```python
from build123d import *

# Parameters (mm, degrees)
SKETCH_1_R          = 2.025
SKETCH_1_R_2        = 13.1
SKETCH_1_R_3        = 3
EXTRUDE_1_DEPTH     = 5
SKETCH_3_R          = 24
CUT_EXTRUDE_2_DEPTH = 10
CUT_EXTRUDE_3_DEPTH = 10
FILLET_1_R          = 3
SKETCH_7_R          = 1.525
CUT_EXTRUDE_4_DEPTH = 10


with BuildPart() as part:
    # 草图1 → 凸台-拉伸1 (new body)
    with BuildSketch(Plane(origin=(0, 0, 0), x_dir=(1, 0, 0), z_dir=(0, 1, 0))):
        with BuildLine():
            Line((76.972140647, 43.13107423), (-4.193547259, 32.732463418))
            ThreePointArc((-4.193547259, 32.732463418), (-32.337515252, -6.579141836), (8.929411765, -31.768940894))
            Line((8.929411765, -31.768940894), (87.705882353, -9.626951786))
            ThreePointArc((87.705882353, -9.626951786), (94.014523475, -4.328783491), (94.205048973, 3.907310252))
            ThreePointArc((94.205048973, 3.907310252), (89.748559809, 18.25955029), (88.242912543, 33.212145922))
            ThreePointArc((88.242912543, 33.212145922), (84.849435117, 40.719066694), (76.972140647, 43.13107423))
        make_face()
        with Locations((0, 17.5)):
            Circle(SKETCH_1_R, mode=Mode.SUBTRACT)
        with Locations((8.75, 15.155444566)):
            Circle(SKETCH_1_R, mode=Mode.SUBTRACT)
        with Locations((-8.75, -15.155444566)):
            Circle(SKETCH_1_R, mode=Mode.SUBTRACT)
        with Locations((0, -17.5)):
            Circle(SKETCH_1_R, mode=Mode.SUBTRACT)
        with Locations((-15.155444566, -8.75)):
            Circle(SKETCH_1_R, mode=Mode.SUBTRACT)
        with Locations((8.75, -15.155444566)):
            Circle(SKETCH_1_R, mode=Mode.SUBTRACT)
        with Locations((15.155444566, -8.75)):
            Circle(SKETCH_1_R, mode=Mode.SUBTRACT)
        with Locations((-17.5, 0)):
            Circle(SKETCH_1_R, mode=Mode.SUBTRACT)
        Circle(SKETCH_1_R_2, mode=Mode.SUBTRACT)
        with Locations((-15.155444566, 8.75)):
            Circle(SKETCH_1_R, mode=Mode.SUBTRACT)
        with Locations((17.5, 0)):
            Circle(SKETCH_1_R, mode=Mode.SUBTRACT)
        with Locations((15.155444566, 8.75)):
            Circle(SKETCH_1_R, mode=Mode.SUBTRACT)
        with Locations((-8.75, 15.155444566)):
            Circle(SKETCH_1_R, mode=Mode.SUBTRACT)
        with Locations((85, 0)):
            Circle(SKETCH_1_R_3, mode=Mode.SUBTRACT)
        with Locations((78.242912543, 33.212145922)):
            Circle(SKETCH_1_R_3, mode=Mode.SUBTRACT)
    extrude(amount=EXTRUDE_1_DEPTH)

    # 草图3 → 切除-拉伸2 (cut)
    with BuildSketch(Plane(origin=(0, 5, 0), x_dir=(1, 0, 0), z_dir=(0, 1, 0))):
        Circle(SKETCH_3_R)
    extrude(amount=-CUT_EXTRUDE_2_DEPTH, mode=Mode.SUBTRACT)

    # 草图4 → 切除-拉伸3 (cut)
    with BuildSketch(Plane(origin=(0, 5, 0), x_dir=(1, 0, 0), z_dir=(0, 1, 0))):
        Polygon((69.770383541, 34.143027562), (75.881597407, 4.105451761), (16.636114037, 27.335685646), align=None)
        with BuildLine():
            ThreePointArc((32, 0), (30.461655113, -9.802426627), (25.994527014, -18.662383699))
            Line((25.994527014, -18.662383699), (76.108728609, -4.576602785))
            Line((76.108728609, -4.576602785), (28.785186198, 13.979021981))
            ThreePointArc((28.785186198, 13.979021981), (31.185942012, 7.171960739), (32, 0))
        make_face()
    extrude(amount=-CUT_EXTRUDE_3_DEPTH, mode=Mode.SUBTRACT)

    # 圆角1
    fillet_1_edges = [part.edges().sort_by_distance(p)[0] for p in [
        (25.994527014, 2.5, 18.662383699),
        (28.785186198, 2.5, -13.979021981),
        (76.108728609, 2.5, 4.576602785),
        (69.770383541, 2.5, -34.143027562),
        (75.881597407, 2.5, -4.105451761),
        (16.636114037, 2.5, -27.335685646),
    ]]
    fillet(fillet_1_edges, radius=FILLET_1_R)

    # 草图7 → 切除-拉伸4 (cut)
    with BuildSketch(Plane.XZ):
        with Locations((0, -27.522163408)):
            Circle(SKETCH_7_R)
        with Locations((33.321534862, -16.496811603)):
            Circle(SKETCH_7_R)
        with Locations((-27.522163408, 0)):
            Circle(SKETCH_7_R)
        with Locations((0, 27.522163408)):
            Circle(SKETCH_7_R)
        with Locations((30.901702525, 21.438107622)):
            Circle(SKETCH_7_R)
        with Locations((56.596303964, -7.370743267)):
            Circle(SKETCH_7_R)
        with Locations((54.969081991, 14.673401739)):
            Circle(SKETCH_7_R)
    extrude(amount=-CUT_EXTRUDE_4_DEPTH, mode=Mode.SUBTRACT)


solid = part.part
```
Verification items for the finished model (mm, model axes). A direction names the side the tool comes from. Round coordinates to 2 decimals unless told otherwise and drop trailing zeros. Order: outer loops, then holes, each group sorted by start corner. A loop starts at its lowest first (then second) coordinate and runs counter-clockwise, first axis right, second up.
1) Cross-section at A-A, the plane x = 51.5. Record the cut outline in (y, z), plus the area to 3 significant figures.
Geometry says:
outline: (0, -39.87) - (5, -39.87) - (5, -31.8) - (0, -31.8) - close; (0, -13.67) - (5, -13.67) - (5, -5.07) - (0, -5.07) - close; (0, 11.49) - (5, 11.49) - (5, 19.8) - (0, 19.8) - close
area: 125 mm2
2) Cross-section at C-C, the plane y = 3.7. Give the number of separate pieces and of enclosed holes in the cut face, plus the area to 3 significant figures.
Geometry says:
separate pieces: 1
enclosed holes: 12
area: 3,810 mm2
3) Cross-section at D-D, the plane x = 14.5. Record the cut outline in (y, z).
Geometry says:
outline: (0, -35.13) - (5, -35.13) - (5, -19.12) - (0, -19.12) - close; (0, 19.12) - (5, 19.12) - (5, 30.2) - (0, 30.2) - close
4) Material ranges on line 1 (Z direction, x = 35, y = 2.6); line 2 (Z direction, x = 0, y = 2.75); line 3 (Z direction, x = 63, y = 4.4), recorded low to high.
Geometry says:
line 1: z = -37.75 to -29.69, -20.14 to -11.54, 16.13 to 24.44
line 2: z = -33.27 to -29.05, -26 to -24, 24 to 26, 29.05 to 33
line 3: z = -41.34 to -33.28, -9.16 to -0.56, 8.26 to 16.57
5) Draft check along Z on faces 3 (the flat face through (47.77, 2.46, 20.85)), 4 (the cylindrical face through (-29.046, 2.465, 0.067)), 5 (the cylindrical face through (-32.48, 2.46, 5.83)), 6 (the flat face through (30, 5, -6)). Enter one of: +Z half, -Z half, draft (parallel to the pull), parting line (faces both ways), or undercut.
Geometry says:
face 3: +Z half
face 4: undercut
face 5: parting line
face 6: draft
6) Cross-section at B-B, the plane x = 0. Record the cut outline in (y, z), plus the area to 3 significant figures.
Geometry says:
outline: (0, -33.27) - (5, -33.27) - (5, -29.05) - (0, -29.05) - close; (0, -26) - (5, -26) - (5, -24) - (0, -24) - close; (0, 24) - (5, 24) - (5, 26) - (0, 26) - close; (0, 29.05) - (5, 29.05) - (5, 33) - (0, 33) - close
area: 60.8 mm2
7) Depth check by flat-ended pin: pin 1 (1 mm diameter, centred on x = 32, y = 1, fed in from -Z). Enter the tip coordinate at first touch or a pass-through.
Geometry says:
pin 1: stops at z = -37.43
8) Tool access check on faces 1 (the cylindrical face through (93.96, 2.46, 4.44)), 2 (the flat face through (72.523, 2.535, -20.614)). Record the directions out of +Z, -Z, +X, -X, +Y, -Y that give a thin tool (end or side, any length) a straight path to the whole face; none if there is none.
Geometry says:
face 1: +X, +Y, -Y
face 2: +Y, -Y
